Could you check a few things on this drawing? It's one solid part, dimensions in mm from its lowest x, y, z. Give positions to 0.01 mm unless a question says otherwise; leave off trailing zeros. Order: outer loops, then holes, each group sorted by start corner. A loop starts at its lowest first (then second) coordinate and runs counter-clockwise, first axis right, second up.
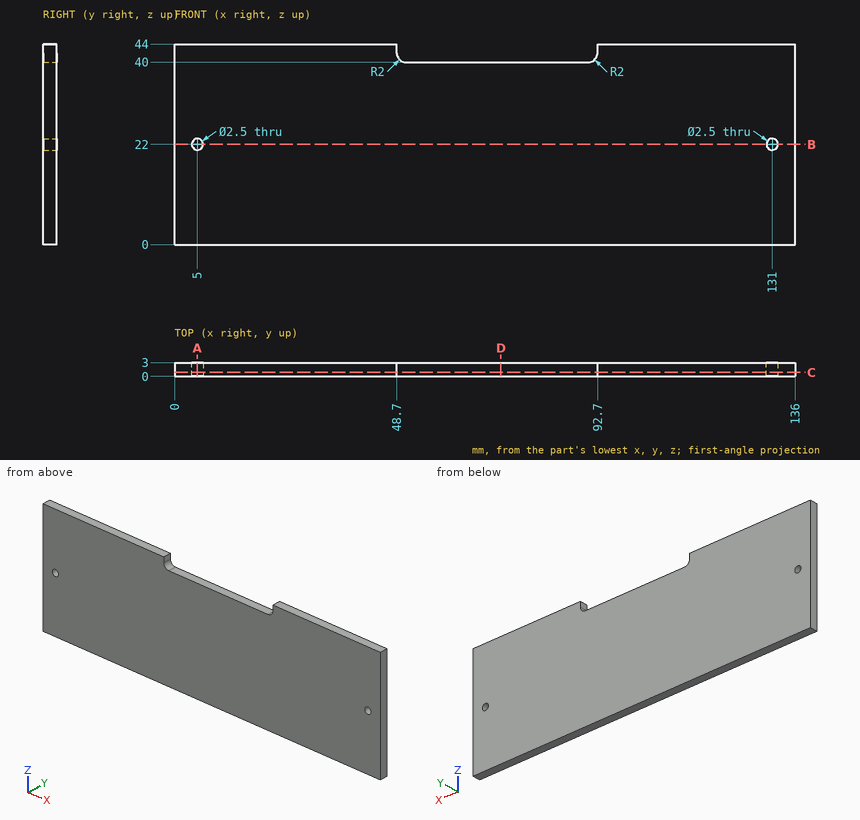
Q1. If we section it at D-D on x = 71.5: List the corners of the cut face in (y, z) for me.
Filled sheet:
outline: (0, 0) - (3, 0) - (3, 40) - (0, 40) - close
Q2. If we section it at A-A on x = 5: List the corners of the cut face in (y, z) for me.
Filled sheet:
outline: (0, 0) - (3, 0) - (3, 20.75) - (0, 20.75) - close; (0, 23.25) - (3, 23.25) - (3, 44) - (0, 44) - close
Q3. I need wall thicknesses on L1, parallel to Z at x = 131, y = 0.95; L2, parallel to Z at x = 78, y = 2.1; L3, parallel to Z at x = 92.5, y = 0.6. Which ranges of each line are inside material? Lowest first, please.
Filled sheet:
L1: z = 0 to 20.75, 23.25 to 44
L2: z = 0 to 40
L3: z = 0 to 41.13
Q4. If we section it at C-C on y = 0.9: List the corners of the cut face in (x, z) for me.
Filled sheet:
outline: (0, 0) - (136, 0) - (136, 44) - (92.7, 44) - (92.7, 42) arc R2 cw to (90.7, 40) - (50.7, 40) arc R2 cw to (48.7, 42) - (48.7, 44) - (0, 44) - close; hole circle Ø2.5 at (5, 22); hole circle Ø2.5 at (131, 22)
Q5. If we section it at B-B on z = 22: List the corners of the cut face in (x, y) for me.
Filled sheet:
outline: (0, 0) - (3.75, 0) - (3.75, 3) - (0, 3) - close; (6.25, 0) - (129.75, 0) - (129.75, 3) - (6.25, 3) - close; (132.25, 0) - (136, 0) - (136, 3) - (132.25, 3) - close
Q6. I'm going to push flat-ended pins straight in: P1, Ø0.6, axis at y = 2, z = 43.5, coming from the -X side; P2, Ø0.9, axis at x = 63, y = 1.5, coming from the +Z side. Where does each tip first touch, or does it pass through?
Filled sheet:
P1: stops at x = 0
P2: stops at z = 40
